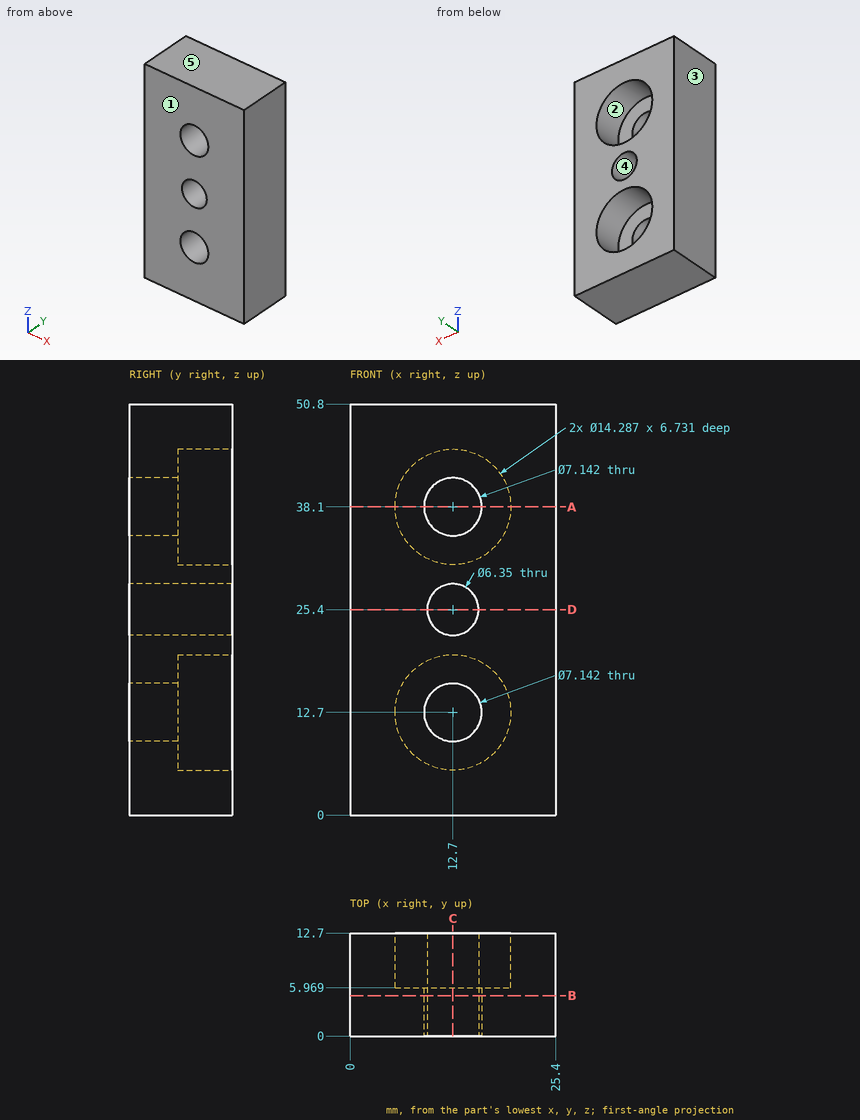
Here's the drawing with two shaded views (mm, measured from the low corner). I have some questions. A direction names the side the tool comes from. Give positions to 0.01 mm unless a question says otherwise; leave off trailing zeros. Order: outer loops, then holes, each group sorted by start corner. A loop starts at its lowest first (then second) coordinate and runs counter-clockwise, first axis right, second up. Notation, with made-up numbers: (39.25, 39.25) - (75.25, 39.25) arc R32 cw to (75.25, 69.25) - close; hole circle Ø9 at (-2.75, 48). An arc over 180 degrees is marked (long way). Use a Markdown table: item, result. Add a question column.
Q1. If we section it at A-A on z = 38.1: Write out the boundary of the cut face in (x, y).
Q2. On a 3-axis mill with a long thin cutter (end or side, diameter ignored), from which of +Z, -Z, +X, -X, +Y, -Y can I reach the whole of each face in a straight line? I mean the marked faces 1 and 2. Say none if no direction works.
Q3. I'm going to push flat-ended pins straight in: pin 1 (5 mm diameter, centred on y = 5, z = 27.5, fed in from -X); pin 2 (7 mm diameter, centred on x = 12.5, z = 15.5, fed in from +Y). Where does each tip first touch, or does it pass through?
Q4. If we section it at D-D on z = 25.4: Write out the boundary of the cut face in (x, y) (1 decimal).
Q5. Please list where these lines run through material, in increasing order: line 1 along Z through (x, y) = (12.7, 1.85) (1 decimal); line 2 along Z through (x, y) = (12.7, 10.75) (1 decimal); line 3 along X through (y, z) = (11, 12.5).
Q6. If we section it at C-C on x = 12.7: Write out the boundary of the cut face in (y, z) (1 decimal).
Q7. If we section it at B-B on y = 5: Count the separate pieces of the cut face and the enclosed holes in it, plus the area to 3 significant figures.
Q8. If we mould it in two halves opening along Z, with no side actions, what happens to the marked faces 3, 4 and 5? For each: released by +Z, released by -Z, zero draft, split by the parting line, or undercut.
Answers follow:
| question | item | result |
|---|---|---|
| 1 | outline | (0, 0) - (9.13, 0) - (9.13, 5.97) - (5.56, 5.97) - (5.56, 12.7) - (0, 12.7) - close; (16.27, 0) - (25.4, 0) - (25.4, 12.7) - (19.84, 12.7) - (19.84, 5.97) - (16.27, 5.97) - close |
| 2 | face 1 | +Z, -Z, +X, -X, -Y |
| 2 | face 2 | +Y |
| 3 | pin 1 | stops at x = 0 |
| 3 | pin 2 | stops at y = 5.97 |
| 4 | outline | (0, 0) - (9.5, 0) - (9.5, 12.7) - (0, 12.7) - close; (15.9, 0) - (25.4, 0) - (25.4, 12.7) - (15.9, 12.7) - close |
| 5 | line 1 | z = 0 to 9.1, 16.3 to 22.2, 28.6 to 34.5, 41.7 to 50.8 |
| 5 | line 2 | z = 0 to 5.6, 19.8 to 22.2, 28.6 to 31, 45.2 to 50.8 |
| 5 | line 3 | x = 0 to 5.56, 19.84 to 25.4 |
| 6 | outline | (0, 0) - (12.7, 0) - (12.7, 5.6) - (6, 5.6) - (6, 9.1) - (0, 9.1) - close; (0, 16.3) - (6, 16.3) - (6, 19.8) - (12.7, 19.8) - (12.7, 22.2) - (0, 22.2) - close; (0, 28.6) - (12.7, 28.6) - (12.7, 31) - (6, 31) - (6, 34.5) - (0, 34.5) - close; (0, 41.7) - (6, 41.7) - (6, 45.2) - (12.7, 45.2) - (12.7, 50.8) - (0, 50.8) - close |
| 7 | separate pieces | 1 |
| 7 | enclosed holes | 3 |
| 7 | area | 1,180 mm^2 |
| 8 | face 3 | zero draft |
| 8 | face 4 | undercut |
| 8 | face 5 | released by +Z |
